from build123d import *

# Parameters (mm, degrees)
CROQUIS1_W              = 240
CROQUIS1_H              = 25
SALIENTE_EXTRUIR1_DEPTH = 50
CROQUIS2_R              = 4.25
CORTAR_EXTRUIR1_DEPTH   = 25
CORTAR_EXTRUIR3_DEPTH   = 26


with BuildPart() as part:
    # Croquis1 → Saliente-Extruir1 (new body)
    with BuildSketch(Plane(origin=(0, 0, 0), x_dir=(1, 0, 0), z_dir=(0, 1, 0))):
        with Locations((0, 2.5)):
            Rectangle(CROQUIS1_W, CROQUIS1_H)
    extrude(amount=-SALIENTE_EXTRUIR1_DEPTH)

    # Croquis2 → Cortar-Extruir1 (cut)
    with BuildSketch(Plane(origin=(0, 0, 0), x_dir=(1, 0, 0), z_dir=(0, 1, 0))):
        with Locations((-70, 2.5)):
            Circle(CROQUIS2_R)
        with Locations((70, 2.5)):
            Circle(CROQUIS2_R)
    extrude(amount=-CORTAR_EXTRUIR1_DEPTH, mode=Mode.SUBTRACT)

    # Croquis3 → Cortar-Extruir3 (cut, through all)
    with BuildSketch(Plane.XY.offset(10)):
        with BuildLine():
            Line((-105, -20.232520372), (-85, -20.232520372))
            ThreePointArc((-85, -20.232520372), (-80.232520372, -25), (-85, -29.767479628))
            Line((-85, -29.767479628), (-105, -29.767479628))
            ThreePointArc((-105, -29.767479628), (-109.767479628, -25), (-105, -20.232520372))
        make_face()
        with BuildLine():
            Line((85, -20.232520372), (105, -20.232520372))
            ThreePointArc((105, -20.232520372), (109.767479628, -25), (105, -29.767479628))
            Line((105, -29.767479628), (85, -29.767479628))
            ThreePointArc((85, -29.767479628), (80.232520372, -25), (85, -20.232520372))
        make_face()
    extrude(amount=-CORTAR_EXTRUIR3_DEPTH, mode=Mode.SUBTRACT)


solid = part.part
Part model, mm, in its own coordinate system. A direction names the side the tool comes from. Coordinates: 2 decimals unless noted, no trailing zeros. Order: outer loops, then holes, each group sorted by start corner. A loop starts at its lowest first (then second) coordinate and runs counter-clockwise, first axis right, second up.
(1) Slice it at C-C, the plane y = -7. Write the cut outline in (x, z), and give its area (3 significant figures).
Check sheet entries:
outline: (-120, -15) - (120, -15) - (120, 10) - (-120, 10) - close; hole circle Ø8.5 at (-70, -2.5); hole circle Ø8.5 at (70, -2.5)
area: 5,890 mm2
(2) Probe L1, parallel to X at y = -18, z = -2.5; L2, parallel to Z at x = 70, y = -19; L3, parallel to Y at x = 87, z = 8.75. List the from-to ranges inside material, lowest first.
Check sheet entries:
L1: x = -120 to -74.25, -65.75 to 65.75, 74.25 to 120
L2: z = -15 to -6.75, 1.75 to 10
L3: y = -50 to -29.77, -20.23 to 0
(3) Slice it at B-B, the plane z = 7.75. Write the cut outline in (x, y), and give its area (3 significant figures).
Check sheet entries:
outline: (-120, -50) - (120, -50) - (120, 0) - (-120, 0) - close; hole (-105, -29.77) - (-85, -29.77) arc R4.77 ccw to (-85, -20.23) - (-105, -20.23) arc R4.77 ccw to start; hole (85, -29.77) - (105, -29.77) arc R4.77 ccw to (105, -20.23) - (85, -20.23) arc R4.77 ccw to start
area: 11,500 mm2
(4) Tool access for faces 1 (the face through (-95, -29.767, -2)), 2 (the face through (74.054, -12.325, -3.777)), 3 (the face through (-2, -25, -15)): list every direction of +Z, -Z, +X, -X, +Y, -Y with a clear straight run to the whole face (end or side of a thin tool).
Check sheet entries:
face 1: +Z, -Z
face 2: +Y
face 3: -Z, +X, -X, +Y, -Y
(5) Slice it at A-A, the plane x = 93. Write the cut outline in (y, z).
Check sheet entries:
outline: (-50, -15) - (-29.77, -15) - (-29.77, 10) - (-50, 10) - close; (-20.23, -15) - (0, -15) - (0, 10) - (-20.23, 10) - close
(6) Pull direction X, two halves, no side cores. Call faces 4 (the face through (70, -25, -3)), 5 (the face through (-120, -25, -2)), 6 (the face through (-2, -50, -3)), 7 (the face through (120, -25, -2)): pulls with the +X half, pulls with the -X half, needs draft (parallel to the pull), parting line crosses it, or undercut.
Check sheet entries:
face 4: undercut
face 5: pulls with the -X half
face 6: needs draft
face 7: pulls with the +X half
(7) Slice it at D-D, the plane z = -2.5. Write the cut outline in (x, y), and give its area (3 significant figures).
Check sheet entries:
outline: (-120, -50) - (120, -50) - (120, 0) - (74.25, 0) - (74.25, -25) - (65.75, -25) - (65.75, 0) - (-65.75, 0) - (-65.75, -25) - (-74.25, -25) - (-74.25, 0) - (-120, 0) - close; hole (-105, -29.77) - (-85, -29.77) arc R4.77 ccw to (-85, -20.23) - (-105, -20.23) arc R4.77 ccw to start; hole (85, -29.77) - (105, -29.77) arc R4.77 ccw to (105, -20.23) - (85, -20.23) arc R4.77 ccw to start
area: 11,100 mm2
